Here's how the part is built. I have some questions about the finished solid (model axes, mm). A direction names the side the tool comes from. Coordinates: 2 decimals unless noted, no trailing zeros. Loops run counter-clockwise (first coordinate to the right, second up) from the corner with the lowest first, then second, coordinate; pieces in that order, holes last. Notation, with made-up numbers: (39, -39) -> (61, -39) arc R27 cw to (61, -6) -> close; hole circle Ø7 at (-35, 88.5). An arc over 180 degrees is marked (long way). Answer as a JSON object with one key per item and string values. Group by question number.
Q1. I want a section at D-D on z = 5. Write out the boundary of the cut face in (x, y), then the cut area to 3 significant figures.
Q2. I want a section at C-C on x = -18.5. Write out the boundary of the cut face in (y, z), then the cut area to 3 significant figures.
Q3. I want a section at B-B on y = 12.5. Write out the boundary of the cut face in (x, z), then the cut area to 3 significant figures.
Q4. Thinking about a two-plate mould opening in X: for faces 1 (the flat face through (-24.5, 0, 3)), 2 (the flat face through (5.101, 0.227, -2)), 3 (the flat face through (-17.5, 0, -1)), which applies, released by +X, released by -X, zero draft, split by the parting line, or undercut?
Q5. I want a section at A-A on x = 20.75. Write out the boundary of the cut face in (y, z), then the cut area to 3 significant figures.
Q6. On a 3-axis mill with a long thin cutter (end or side, diameter ignored), from which of +Z, -Z, +X, -X, +Y, -Y can I reach the whole of each face in a straight line? I mean faces 4 (the flat face through (24.5, 0, 3)), 5 (the flat face through (-3, 0, -0.6)), 6 (the flat face through (0, 16.25, 3)), 7 (the flat face through (-20, 10, -1)), 8 (the flat face through (0, 0, 0)). Say none if no direction works.
Q7. I need wall thicknesses on line 1 (X direction, y = 12.5, z = -0.85); line 2 (X direction, y = 4, z = -1); line 3 (Y direction, x = -20.75, z = -1.55). Which ranges of each line are inside material? Lowest first, please.
Q8. I'm going to push flat-ended pins straight in: pin 1 (6 mm diameter, centred on x = 15.5, y = -11, fed in from +Z); pin 2 (0.9 mm diameter, centred on x = 20.75, y = 12.5, fed in from +Z); pin 3 (3 mm diameter, centred on x = 1, y = -3.5, fed in from -Z); pin 4 (4 mm diameter, centred on x = -20, y = 12, fed in from +Z). Where does each tip first touch, or does it pass through?
Solid Edge part; units mm, degrees
sketch "Sketch1" plane through (0, 0, 0) normal (0, 0, 1) x (1, 0, 0)
  line L0 (-24.5, 16.25) -> (-24.5, -16.25)
  line L1 (-24.5, -16.25) -> (24.5, -16.25)
  line L2 (24.5, -16.25) -> (24.5, 16.25)
  line L3 (24.5, 16.25) -> (-24.5, 16.25)
extrude "Protrusion1" add sketch "Sketch1" against normal blind 2
sketch "Sketch2" plane through (0, 0, 0) normal (0, 0, 1) x (1, 0, 0)
  line L0 (-23.5, 15.25) -> (-23.5, -15.25)
  line L1 (-23.5, -15.25) -> (23.5, -15.25)
  line L2 (23.5, -15.25) -> (23.5, 15.25)
  line L3 (23.5, 15.25) -> (-23.5, 15.25)
  line L4 (-24.5, 16.25) -> (-24.5, -16.25)
  line L5 (-24.5, -16.25) -> (24.5, -16.25)
  line L6 (24.5, -16.25) -> (24.5, 16.25)
  line L7 (24.5, 16.25) -> (-24.5, 16.25)
extrude "ExtrudedProtrusion_2" add sketch "Sketch2" along normal blind 8.5
sketch "Sketch3" plane through (0, 0, 0) normal (0, 0, 1) x (1, 0, 0)
  line L0 (-17.5, -10) -> (-17.5, 10)
  line L1 (-17.5, 10) -> (-23.5, 10)
  line L2 (-23.5, 10) -> (-23.5, -10)
  line L3 (-23.5, -10) -> (-17.5, -10)
extrude "Cutout1" cut sketch "Sketch3" against normal up to vertex (2 mm away)
sketch "Sketch4" plane through (0, 0, 0) normal (0, 0, 1) x (1, 0, 0)
  circle A0 centre (-20.75, 12.5) radius 0.75
  circle A1 centre (-20.75, -12.5) radius 0.75
  circle A2 centre (20.75, -12.5) radius 0.75
  circle A3 centre (20.75, 12.5) radius 0.75
extrude "Cutout2" cut sketch "Sketch4" against normal up to vertex (2 mm away)
sketch "Sketch5" plane through (0, 0, -2) normal (0, 0, -1) x (1, 0, 0)
  line L0 (-10.05, 5.5) -> (-10.05, -4.5)
  line L1 (-10.05, -4.5) -> (4.7, -4.5)
  line L2 (4.7, -4.5) -> (4.7, 5.5)
  line L3 (4.7, 5.5) -> (-10.05, 5.5)
extrude "ExtrudedCutout_4" cut sketch "Sketch5" against normal blind 1
sketch "Sketch6" plane through (0, 0, -2) normal (0, 0, -1) x (1, 0, 0)
  line L0 (4.7, 5.5) -> (-10.05, 5.5)
  line L1 (-10.05, 5.5) -> (-10.05, -4.5)
  line L2 (-10.05, -4.5) -> (4.7, -4.5)
  line L3 (4.7, -4.5) -> (4.7, 5.5)
extrude "Protrusion2" add sketch "Sketch6" against normal up to vertex (1 mm away)
sketch "Sketch7" plane through (0, 0, -2) normal (0, 0, -1) x (1, 0, 0)
  line L0 (-10.05, -5) -> (4.7, -5)
  line L1 (4.7, -5) -> (4.7, 5)
  line L2 (4.7, 5) -> (-10.05, 5)
  line L3 (-10.05, 5) -> (-10.05, -5)
extrude "ExtrudedCutout_5" cut sketch "Sketch7" against normal blind 1
sketch "Sketch8" plane through (0, 0, -2) normal (0, 0, -1) x (1, 0, 0)
  line L0 (4.95, 5.25) -> (-10.3, 5.25)
  line L1 (-10.3, 5.25) -> (-10.3, -5.25)
  line L2 (-10.3, -5.25) -> (4.95, -5.25)
  line L3 (4.95, -5.25) -> (4.95, 5.25)
extrude "ExtrudedCutout_6" cut sketch "Sketch8" against normal blind 1.4
sketch "Sketch9" plane through (0, 0, 0) normal (0, 0, 1) x (-1, 0, 0)
  circle A0 centre (20.75, 12.5) radius 1.75
  circle A1 centre (20.75, 12.5) radius 0.75
  circle A2 centre (20.75, -12.5) radius 1.75
  circle A3 centre (20.75, -12.5) radius 0.75
  circle A4 centre (-20.75, -12.5) radius 1.75
  circle A5 centre (-20.75, -12.5) radius 0.75
  circle A6 centre (-20.75, 12.5) radius 1.75
  circle A7 centre (-20.75, 12.5) radius 0.75
extrude "ExtrudedProtrusion_6" add sketch "Sketch9" along normal blind 1.1
properties material "Graphite"
Result set:
{
 "1": {"outline": "(-24.5, -16.25) -> (24.5, -16.25) -> (24.5, 16.25) -> (-24.5, 16.25) -> close; hole (-23.5, -15.25) -> (23.5, -15.25) -> (23.5, 15.25) -> (-23.5, 15.25) -> close", "area": "159 mm²"},
 "2": {"outline": "(-16.25, -2) -> (-10, -2) -> (-10, 0) -> (-15.25, 0) -> (-15.25, 8.5) -> (-16.25, 8.5) -> close; (10, -2) -> (16.25, -2) -> (16.25, 8.5) -> (15.25, 8.5) -> (15.25, 0) -> (10, 0) -> close", "area": "42.0 mm²"},
 "3": {"outline": "(-24.5, -2) -> (-21.5, -2) -> (-21.5, 1.1) -> (-22.5, 1.1) -> (-22.5, 0) -> (-23.5, 0) -> (-23.5, 8.5) -> (-24.5, 8.5) -> close; (-20, -2) -> (20, -2) -> (20, 1.1) -> (19, 1.1) -> (19, 0) -> (-19, 0) -> (-19, 1.1) -> (-20, 1.1) -> close; (21.5, -2) -> (24.5, -2) -> (24.5, 8.5) -> (23.5, 8.5) -> (23.5, 0) -> (22.5, 0) -> (22.5, 1.1) -> (21.5, 1.1) -> close", "area": "113 mm²"},
 "4": {"face 1": "released by -X", "face 2": "zero draft", "face 3": "undercut"},
 "5": {"outline": "(-16.25, -2) -> (-13.25, -2) -> (-13.25, 1.1) -> (-14.25, 1.1) -> (-14.25, 0) -> (-15.25, 0) -> (-15.25, 8.5) -> (-16.25, 8.5) -> close; (-11.75, -2) -> (11.75, -2) -> (11.75, 1.1) -> (10.75, 1.1) -> (10.75, 0) -> (-10.75, 0) -> (-10.75, 1.1) -> (-11.75, 1.1) -> close; (13.25, -2) -> (16.25, -2) -> (16.25, 8.5) -> (15.25, 8.5) -> (15.25, 0) -> (14.25, 0) -> (14.25, 1.1) -> (13.25, 1.1) -> close", "area": "80.4 mm²"},
 "6": {"face 4": "+Z, -Z, +X, +Y, -Y", "face 5": "-Z", "face 6": "+Z, -Z, +X, -X, +Y", "face 7": "+Z, -Z", "face 8": "+Z"},
 "7": {"line 1": "x = -24.5 to -21.5, -20 to 20, 21.5 to 24.5", "line 2": "x = -24.5 to -23.5, -17.5 to -10.3, 4.95 to 24.5", "line 3": "y = -16.25 to -13.25, -11.75 to -10, 10 to 11.75, 13.25 to 16.25"},
 "8": {"pin 1": "stops at z = 0", "pin 2": "passes through", "pin 3": "stops at z = -0.6", "pin 4": "stops at z = 1.1"}
}
